```python
from build123d import *

# Parameters (mm, degrees)
SKETCH1_R               = 50
BOSS_EXTRUDE1_DEPTH     = 250
CUT_EXTRUDE1_DEPTH      = 260.807621135
CUT_EXTRUDE1_DEPTH_BACK = 260.807621135
SKETCH3_W               = 7.515334491
SKETCH3_H               = 262.678834124


with BuildPart() as part:
    # Sketch1 → Boss-Extrude1 (new body)
    with BuildSketch(Plane(origin=(0, 0, 0), x_dir=(1, 0, 0), z_dir=(0, 1, 0))):
        with Locations(Location((0, 0, 0), (0, 0, 270))):
            Circle(SKETCH1_R)
    extrude(amount=BOSS_EXTRUDE1_DEPTH)

    # Sketch2 → Cut-Revolve1 (revolve, cut)
    with BuildSketch(Plane.XY):
        with BuildLine():
            Line((0, 300), (0, 200))
            ThreePointArc((0, 200), (50, 250), (0, 300))
        make_face()
    cut_revolve1 = revolve(axis=Axis((0, 300, 0), (0, -1, 0)), mode=Mode.SUBTRACT)

    # Mirror2: Cut-Revolve1 across plane
    add(cut_revolve1.mirror(Plane.ZX.offset(125)), mode=Mode.SUBTRACT)

    # Sketch3 → Cut-Extrude1 (cut, two sides: drawn at the far end of the back side and taken through both)
    with BuildSketch(Plane.XY.offset(-CUT_EXTRUDE1_DEPTH_BACK)):
        with Locations((47.239245373, 124.642126929)):
            Rectangle(SKETCH3_W, SKETCH3_H)
    extrude(amount=CUT_EXTRUDE1_DEPTH + CUT_EXTRUDE1_DEPTH_BACK, mode=Mode.SUBTRACT)


solid = part.part
```
Geometry: final body of the model. Coordinates: model frame, mm. Coordinates: 2 decimals unless noted, no trailing zeros. Order: outer loops, then holes, each group sorted by start corner. A loop starts at its lowest first (then second) coordinate and runs counter-clockwise, first axis right, second up.
Item 1: Section query A-A (y = 169). Output: boundary loops of the cut face in (x, z).
Answer:
outline: (43.48, -24.69) - (43.48, 24.69) arc R50 ccw (long way) to start
Item 2: Material intervals for line 1 along Z through (x, y) = (-15, 214); line 2 along Z through (x, y) = (-19.5, 208.5); line 3 along X through (y, z) = (27, 5.5), sorted ascending.
Answer:
line 1: z = -47.7 to -31.29, 31.29 to 47.7
line 2: z = -46.04 to -19.94, 19.94 to 46.04
line 3: x = -49.7 to -41.72, 41.72 to 43.48
Item 3: Section query D-D (y = 209.5). Output: boundary loops of the cut face in (x, z), then the cut area to 3 significant figures.
Answer:
outline: (43.48, -24.69) - (43.48, 24.69) arc R50 ccw (long way) to start; hole circle Ø58.64 at (0, 0)
area: 4,940 mm2
Item 4: Section query C-C (z = 40.5). Output: boundary loops of the cut face in (x, y), then the cut area to 3 significant figures.
Answer:
outline: (-29.32, 0) arc R29.32 cw to (29.32, 0) - (29.32, 250) arc R29.32 cw to (-29.32, 250) - close
area: 12,000 mm2
Item 5: Contact query for flat-ended pins moving along their axis: P1, Ø10, axis at x = 17, z = -3, coming from the +Y side; P2, Ø1, axis at x = 7, y = 44, coming from the +Z side; P3, Ø5, axis at x = -30.5, y = 198, coming from the -Z side. Output: stop coordinate, or through.
Answer:
P1: stops at y = 205.23
P2: stops at z = 49.58
P3: stops at z = -41.42
Item 6: Section query B-B (x = 0). Output: boundary loops of the cut face in (y, z).
Answer:
outline: (0, -50) - (250, -50) arc R50 cw to (250, 50) - (0, 50) arc R50 cw to start
